Autodesk Inventor part; units mm, degrees
ref_plane "YZ Plane" through (0, 0, 0) normal (1, 0, 0) x (0, 1, 0)
ref_plane "XZ Plane" through (0, 0, 0) normal (0, 1, 0) x (-1, 0, 0)
ref_plane "XY Plane" through (0, 0, 0) normal (0, 0, 1) x (1, 0, 0)
sketch "Sketch1" plane through (0, 0, 0) normal (0, 1, 0) x (-1, 0, 0)
  line L0 (0, 0) -> (60, 0)
  line L1 (60, 0) -> (60, -30)
  line L2 (60, -30) -> (0, -30)
  line L3 (0, -30) -> (0, 0)
  dimension "d0" = 60
  dimension "d1" = 30
extrude "Extrusion1" add sketch "Sketch1" along normal blind 5
sketch "Sketch2" plane through (0, 5, 0) normal (0, 1, 0) x (1, 0, 0)
  line L0 (-60, 30) -> (-60, 0)
  line L1 (0, 30) -> (-60, 30)
  line L2 (-60, 0) -> (-55, 0)
  line L3 (-55, 0) -> (-55, 30)
  line L4 (-55, 30) -> (-60, 30)
  line L5 (-60, 30) -> (-60, 0)
  point P0 (0, 0)
  dimension "d4" = 5
extrude "Extrusion2" add sketch "Sketch2" along normal blind 10
sketch "Sketch3" plane through (0, 0, 0) normal (0, -1, 0) x (1, 0, 0)
  line L0 (0, -30) -> (-60, -30)
  line L1 (0, 0) -> (-5, 0)
  line L2 (-5, 0) -> (-5, -30)
  line L3 (-5, -30) -> (0, -30)
  line L4 (0, -30) -> (0, 0)
  dimension "d7" = 5
extrude "Extrusion3" add sketch "Sketch3" along normal blind 59
sketch "Sketch4" plane through (0, 5, 0) normal (1, 0, 0) x (0, 0, -1)
  line L0 (0, -64) -> (30, -64)
  circle A0 centre (15, -49) radius 6.5
  point P0 (0, -5)
  dimension "d11" = 13
extrude "Extrusion4" cut sketch "Sketch4" against normal up to surface (5 mm away)
properties part number "Bracket_Support_2"
Can you work these out from the model? Positions are in its coordinate system, mm. A direction names the side the tool comes from. Round coordinates to 2 decimals unless told otherwise and drop trailing zeros. Loops run counter-clockwise (first coordinate to the right, second up) from the corner with the lowest first, then second, coordinate; pieces in that order, holes last. Notation, with made-up numbers: M 89.25,50.25 L 93.25,50.25 A21 ccw 93.25,64.25 Z; hole C -3,5 d5. An arc over 180 degrees is marked long. Answer as a JSON object with one key per item and string values. Group by question number.
Q1. Will these pins go through, and if not, where does the flat tip stop? pin 1 (9 mm diameter, centred on x = -23, z = -17, fed in from +Y); pin 2 (6 mm diameter, centred on x = -17.5, z = -13.5, fed in from -Y); pin 3 (3 mm diameter, centred on y = 11, z = -14.5, fed in from +X); pin 4 (12 mm diameter, centred on x = -13.5, y = -10, fed in from -Z).
Q2. Imagine slicing it at D-D, the plane z = -19. Please give me the cut outline in (x, y).
Q3. Imagine slicing it at A-A, the plane z = -15. Please give me the cut outline in (x, y), then the cut area to 3 significant figures.
Q4. Imagine slicing it at C-C, the plane x = -11.5. Please give me the cut outline in (y, z).
Q5. Imagine slicing it at B-B, the plane y = -44. Please give me the cut outline in (x, z), then the cut area to 3 significant figures.
Q6. Please list where these lines run through material, in increasing order: L1, parallel to Y at x = -3.05, z = -15; L2, parallel to X at y = -8, z = -25; L3, parallel to Y at x = -25.5, z = -21.75.
Q7. On a 3-axis mill with a long thin cutter (end or side, diameter ignored), from which of +Z, -Z, +X, -X, +Y, -Y can I reach the whole of each face in a straight line? I mean faces 1 (the flat face through (-32, 0, -15)), 2 (the flat face through (-55, 10, -15)), 3 (the flat face through (-3, -59, -15)). Say none if no direction works.
Q8. We'd pull the mould along Z, two halves only. Please class faces 4 (the cylindrical face through (-2.465, -47.955, -9.842)), 5 (the flat face through (-60, 7, -15)), 6 (the flat face through (-21, 3, -30)): +Z half, -Z half, draft (parallel to the pull), parting line (faces both ways), or undercut.
Findings:
{
 "1": {"pin 1": "stops at y = 5", "pin 2": "stops at y = 0", "pin 3": "stops at x = -55", "pin 4": "passes through"},
 "2": {"outline": "M -60,0 L -5,0 L -5,-38.88 L 0,-38.88 L 0,5 L -55,5 L -55,15 L -60,15 Z; M -5,-59 L 0,-59 L 0,-49.12 L -5,-49.12 Z"},
 "3": {"outline": "M -60,0 L -5,0 L -5,-37.5 L 0,-37.5 L 0,5 L -55,5 L -55,15 L -60,15 Z; M -5,-59 L 0,-59 L 0,-50.5 L -5,-50.5 Z", "area": "580 mm2"},
 "4": {"outline": "M 0,-30 L 5,-30 L 5,0 L 0,0 Z"},
 "5": {"outline": "M -5,-30 L 0,-30 L 0,-21.5 L -5,-21.5 Z; M -5,-8.5 L 0,-8.5 L 0,0 L -5,0 Z", "area": "85.0 mm2"},
 "6": {"L1": "y = -59 to -50.5, -37.5 to 5", "L2": "x = -5 to 0", "L3": "y = 0 to 5"},
 "7": {"face 1": "+Z, -Z, -X, -Y", "face 2": "+Z, -Z, +X, +Y", "face 3": "+Z, -Z, +X, -X, -Y"},
 "8": {"face 4": "undercut", "face 5": "draft", "face 6": "-Z half"}
}
